Design review of the part built by this model. Coordinates are the model's own, in mm. A direction names the side the tool comes from. Round coordinates to 2 decimals unless told otherwise and drop trailing zeros. Order: outer loops, then holes, each group sorted by start corner. A loop starts at its lowest first (then second) coordinate and runs counter-clockwise, first axis right, second up.
from build123d import *

# Parameters (mm, degrees)
SKETCH1_W           = 54.61
SKETCH1_H           = 30.48
BOSS_EXTRUDE1_DEPTH = 2.54
FILLET1_R           = 2.54
BOSS_EXTRUDE2_DEPTH = 6.35
SKETCH3_W           = 6.35
SKETCH3_H           = 6.35
CUT_EXTRUDE1_DEPTH  = 12.7
SKETCH4_R           = 1.397
CUT_EXTRUDE2_DEPTH  = 14.9700001


with BuildPart() as part:
    # Sketch1 → Boss-Extrude1 (new body)
    with BuildSketch(Plane(origin=(0, 0, 0), x_dir=(1, 0, 0), z_dir=(0, 1, 0))):
        Rectangle(SKETCH1_W, SKETCH1_H)
    extrude(amount=-BOSS_EXTRUDE1_DEPTH)

    # Fillet1
    fillet1_edges = [part.edges().sort_by_distance(p)[0] for p in [
        (27.305, -1.27, 15.24),
        (-27.305, -1.27, 15.24),
        (-27.305, -1.27, -15.24),
        (27.305, -1.27, -15.24),
    ]]
    fillet(fillet1_edges, radius=FILLET1_R)

    # Sketch2 → Boss-Extrude2 (add, symmetric)
    with BuildSketch(Plane.XY):
        with BuildLine():
            add(Edge.make_bspline(
                [(34.925, -13.97), (32.641767313, -4.413096047), (27.305, 0)],
                knots=[0, 0, 0, 0.368203859, 0.368203859, 0.368203859], degree=2))
            Line((27.305, 0), (27.305, -13.97))
            Line((27.305, -13.97), (34.925, -13.97))
        make_face()
    boss_extrude2 = extrude(amount=BOSS_EXTRUDE2_DEPTH, both=True)

    # Sketch3 → Cut-Extrude1 (cut)
    with BuildSketch(Plane(origin=(0, 0, 0), x_dir=(1, 0, 0), z_dir=(0, 1, 0))):
        with Locations((31.75, 0)):
            Rectangle(SKETCH3_W, SKETCH3_H)
    cut_extrude1 = extrude(amount=-CUT_EXTRUDE1_DEPTH, mode=Mode.SUBTRACT)

    # Sketch4 → Cut-Extrude2 (cut, through all)
    with BuildSketch(Plane(origin=(0, -13.97, 0), x_dir=(-1, 0, 0), z_dir=(0, -1, 0))):
        with Locations((-30.607, 0)):
            Circle(SKETCH4_R)
    cut_extrude2 = extrude(amount=-CUT_EXTRUDE2_DEPTH, mode=Mode.SUBTRACT)

    # Mirror1: Boss-Extrude2, Cut-Extrude1, Cut-Extrude2 across plane
    add(boss_extrude2.mirror(Plane(origin=(0, 0, 0), x_dir=(0, 0, 1), z_dir=(1, 0, 0))))
    add(cut_extrude1.mirror(Plane(origin=(0, 0, 0), x_dir=(0, 0, 1), z_dir=(1, 0, 0))), mode=Mode.SUBTRACT)
    add(cut_extrude2.mirror(Plane(origin=(0, 0, 0), x_dir=(0, 0, 1), z_dir=(1, 0, 0))), mode=Mode.SUBTRACT)


solid = part.part
1) To check wall thickness, follow line 1 along X through (y, z) = (-13.3, 0) (3 decimals); line 2 along X through (y, z) = (-10.5, 2) (3 decimals); line 3 along Y through (x, z) = (3.5, 9). State the ranges of each line that lie inside material, in increasing order.
Results:
line 1: x = -34.76 to -32.004, -29.21 to -27.305, 27.305 to 29.21, 32.004 to 34.76
line 2: x = -28.575 to -27.305, 27.305 to 28.575
line 3: y = -2.54 to 0
2) For faces 4 (the face through (28.575, -7, 0)), 5 (the face through (-28.575, -7, 0)), 6 (the face through (-27.305, -8, 0)), 7 (the face through (26.541, -1.288, 14.516)), list the 3-axis set-ups (+Z, -Z, +X, -X, +Y, -Y) from which the entire face can be reached by the end or side of a thin tool; tool diameter is ignored.
Results:
face 4: +X, +Y
face 5: -X, +Y
face 6: +Z, -Z, -Y
face 7: +Z, +X, +Y, -Y
3) Clearance check with flat-ended pins moving along their axes: P1, Ø3, axis at x = -30, y = -7, coming from the +Z side; P2, Ø5.5, axis at y = -10.5, z = 3, coming from the +X side; P3, Ø5, axis at x = 30.5, y = -9, coming from the -Z side; P4, Ø1, axis at y = -10, z = -8.5, coming from the +X side. State where each tip first meets the part, or that it passes through.
Results:
P1: stops at z = 6.35
P2: stops at x = 34.75
P3: stops at z = -6.35
P4: passes through
4) Take a section at B-B on x = -13. Give the boundary of the cut face in (y, z), plus the area to 3 significant figures.
Results:
outline: (-2.54, -15.24) - (0, -15.24) - (0, 15.24) - (-2.54, 15.24) - close
area: 77.4 mm2
5) The part is to be moulded in two halves that separate along Z. For faces 1 (the face through (-27.305, -1, -9)), 2 (the face through (-30, -8, -6.35)), 3 (the face through (29.275, -13.344, -0.42)), say which applies: released by +Z, released by -Z, zero draft, split by the parting line, or undercut.
Results:
face 1: zero draft
face 2: released by -Z
face 3: undercut
6) Take a section at A-A on z = -7. Give the boundary of the cut face in (x, y) (3 decimals).
Results:
outline: (-27.305, -2.54) - (27.305, -2.54) - (27.305, 0) - (-27.305, 0) - close
